Answer from the drawing. Dimensions are ordinates in mm from the lowest x, y and z of the part. Give positions to 0.01 mm unless a question says otherwise; leave off trailing zeros. Loops run counter-clockwise (first coordinate to the right, second up) from the corner with the lowest first, then second, coordinate; pieces in that order, holes last. Notation, with made-up numbers: M 26,11.5 L 82,11.5 A27 cw 82,29.5 Z; hole C -10,-31 d8. An arc over 180 degrees is marked long. Use a Markdown table: item, result.
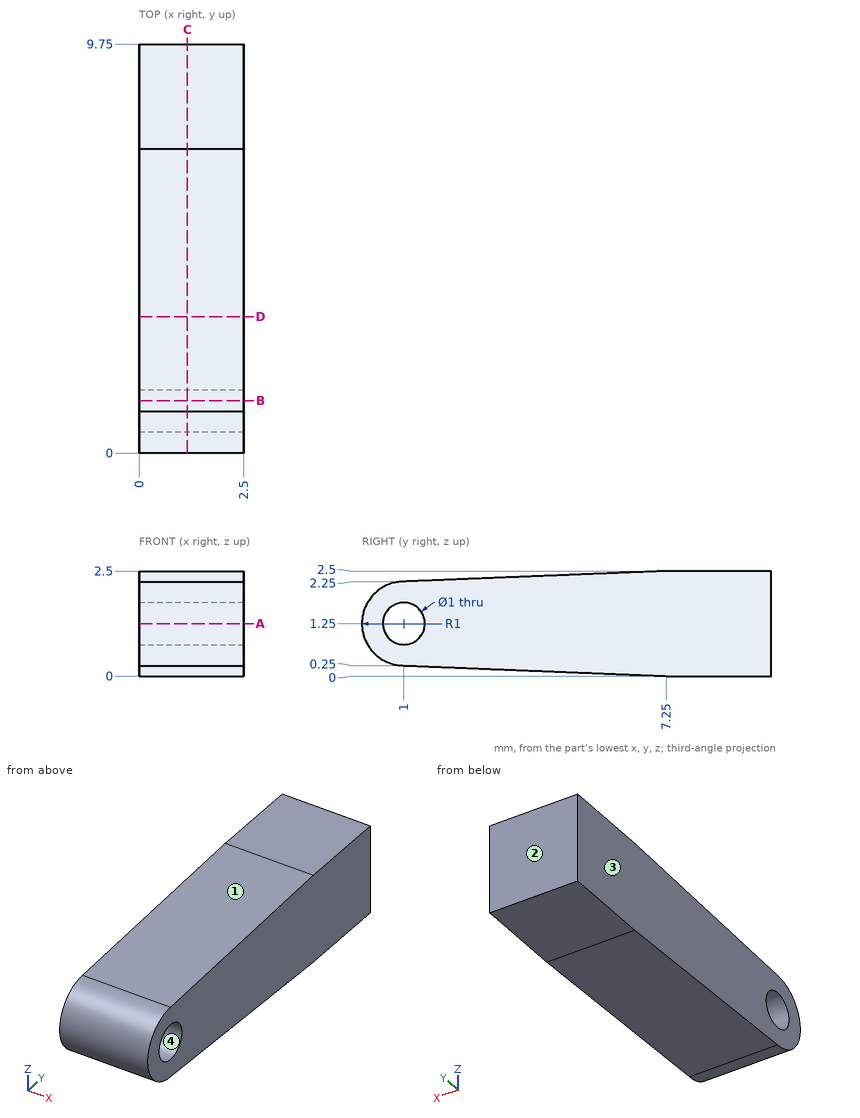
(1) Consider probe 1 along Y at (x, z) = (1.1, 1.25); probe 2 along Z at (x, y) = (1.9, 2.5); probe 3 along Z at (x, y) = (0.55, 6). Determine where each line is inside the solid, lowest interval first. Write a range as [from, to].
Entries:
| item | result |
|---|---|
| probe 1 | y = [0, 0.5], [1.5, 9.75] |
| probe 2 | z = [0.19, 2.31] |
| probe 3 | z = [0.05, 2.45] |
(2) A cutting plane is placed at D-D (y = 3.25). Write down the section's boundary in (x, z), and give its area (3 significant figures).
Entries:
| item | result |
|---|---|
| outline | M 0,0.16 L 2.5,0.16 L 2.5,2.34 L 0,2.34 Z |
| area | 5.45 mm² |
(3) The mould has two halves that part along Y. Classify the marked faces 1, 2, 3 and 4: released by +Y, released by -Y, zero draft, split by the parting line, or undercut.
Entries:
| item | result |
|---|---|
| face 1 | released by -Y |
| face 2 | released by +Y |
| face 3 | zero draft |
| face 4 | undercut |
(4) A cutting plane is placed at C-C (x = 1.15). Write down the section's boundary in (y, z), and give its area (3 significant figures).
Entries:
| item | result |
|---|---|
| outline | M 1,0.25 L 7.25,0 L 9.75,0 L 9.75,2.5 L 7.25,2.5 L 1,2.25 A1 ccw Z; hole C 1,1.25 d1 |
| area | 21.1 mm² |
(5) A cutting plane is placed at A-A (z = 1.25). Write down the section's boundary in (x, y), and give its area (3 significant figures).
Entries:
| item | result |
|---|---|
| outline | M 0,0 L 2.5,0 L 2.5,0.5 L 0,0.5 Z; M 0,1.5 L 2.5,1.5 L 2.5,9.75 L 0,9.75 Z |
| area | 21.9 mm² |
(6) A cutting plane is placed at B-B (y = 1.25). Write down the section's boundary in (x, z), and give its area (3 significant figures).
Entries:
| item | result |
|---|---|
| outline | M 0,0.24 L 2.5,0.24 L 2.5,0.82 L 0,0.82 Z; M 0,1.68 L 2.5,1.68 L 2.5,2.26 L 0,2.26 Z |
| area | 2.88 mm² |
